Verification items for the finished model (mm, model axes). A direction names the side the tool comes from. Round coordinates to 2 decimals unless told otherwise and drop trailing zeros. Loops run counter-clockwise (first coordinate to the right, second up) from the corner with the lowest first, then second, coordinate; pieces in that order, holes last. Notation, with made-up numbers: (-12, 44) -> (3, 44) arc R17 ccw to (3, 62) -> close; hole circle Ø9 at (-4.5, -38). An arc over 180 degrees is marked (long way). Write item = value, one per line. Start each with the question number.
```python
from build123d import *

# Parameters (mm, degrees)
F0_W     = 11
F0_H     = 22
F0_R     = 0.5
F1_DEPTH = 15
F0_H_2   = 5
F0_R_2   = 1
F2_DEPTH = 1.5
F3_DEPTH = 7


with BuildPart() as f1:
    # F0 (on Top) → F1 (new body)
    with BuildSketch(Plane.XY):
        Rectangle(F0_W, F0_H)
        with Locations((0, -5)):
            Circle(F0_R, mode=Mode.SUBTRACT)
        with Locations((0, -5)):
            Circle(F0_R)
    extrude(amount=F1_DEPTH)

    # F0 (on Top) → F2 (join)
    with BuildSketch(Plane.XY):
        with Locations((0, -13.5)):
            Rectangle(F0_W, F0_H_2)
        with Locations((0, -14.5)):
            Circle(F0_R_2, mode=Mode.SUBTRACT)
        with Locations((0, 13.5)):
            Rectangle(F0_W, F0_H_2)
        with Locations((0, 14.5)):
            Circle(F0_R_2, mode=Mode.SUBTRACT)
    extrude(amount=-F2_DEPTH)

    # F0 (on Top) → F3 (join)
    with BuildSketch(Plane.XY):
        Rectangle(F0_W, F0_H)
        with Locations((0, -5)):
            Circle(F0_R, mode=Mode.SUBTRACT)
    extrude(amount=-F3_DEPTH)


solid = f1.part
```
(1) Section check C-C on y = -5. Enter the section's corners in (x, z), then the cut area to 3 significant figures.
(2) Depth check by flat-ended pin: pin 1 Ø3.5 at (x, z) = (-2, 8.5) entering from +Y; pin 2 Ø0.8 at (x, y) = (0, -5) entering from -Z; pin 3 Ø1.5 at (x, y) = (0.5, -13.5) entering from -Z; pin 4 Ø1.2 at (x, y) = (0, -14.5) entering from -Z. Enter the tip coordinate at first touch or a pass-through.
(3) Section check D-D on x = 1.5. Enter the section's corners in (y, z).
(4) Draft check along X on faces 1 (the cylindrical face through (-0.065, -4.504, -3.451)), 2 (the flat face through (0, -13, -1.5)), 3 (the flat face through (5.5, 0, 4)), 4 (the flat face through (-5.5, 0, 4)). Enter one of: +X half, -X half, draft (parallel to the pull), parting line (faces both ways), or undercut.
(5) Section check A-A on x = 0. Enter the section's corners in (y, z), then the cut area to 3 significant figures.
(6) Access from +Z, -Z, +X, -X, +Y, -Y to the whole of each face (thin tool, end or side, straight path). Record for faces 5 (the flat face through (0, 11, -4)), 6 (the flat face through (0, -11, -4)), 7 (the flat face through (0, -5, 0)), 8 (the flat face through (0, 11, 7)), 9 (the flat face through (0, -11, 7)).
(7) Section check B-B on y = 14.5. Enter the section's corners in (x, z).
(8) Scan lines: line 1 (Y direction, x = 0, z = -0.8); line 2 (Y direction, x = 0, z = -4.25); line 3 (Y direction, x = -3.5, z = -5). Record each from-to range of solid material in increasing order. Write a range as [from, to].
Computed values:
q1.outline = (-5.5, -7) -> (-0.5, -7) -> (-0.5, 0) -> (0.5, 0) -> (0.5, -7) -> (5.5, -7) -> (5.5, 15) -> (-5.5, 15) -> close
q1.area = 235 mm²
q2.pin_1 = 11
q2.pin_2 = 0
q2.pin_3 = -1.5
q2.pin_4 = through
q3.outline = (-16, -1.5) -> (-11, -1.5) -> (-11, -7) -> (11, -7) -> (11, -1.5) -> (16, -1.5) -> (16, 0) -> (11, 0) -> (11, 15) -> (-11, 15) -> (-11, 0) -> (-16, 0) -> close
q4.face_1 = undercut
q4.face_2 = draft
q4.face_3 = +X half
q4.face_4 = -X half
q5.outline = (-16, -1.5) -> (-15.5, -1.5) -> (-15.5, 0) -> (-16, 0) -> close; (-13.5, -1.5) -> (-11, -1.5) -> (-11, -7) -> (-5.5, -7) -> (-5.5, 0) -> (-4.5, 0) -> (-4.5, -7) -> (11, -7) -> (11, -1.5) -> (13.5, -1.5) -> (13.5, 0) -> (11, 0) -> (11, 15) -> (-11, 15) -> (-11, 0) -> (-13.5, 0) -> close; (15.5, -1.5) -> (16, -1.5) -> (16, 0) -> (15.5, 0) -> close
q5.area = 486 mm²
q6.face_5 = -Z, +X, -X, +Y
q6.face_6 = -Z, +X, -X, -Y
q6.face_7 = -Z
q6.face_8 = +Z, +X, -X, +Y
q6.face_9 = +Z, +X, -X, -Y
q7.outline = (-5.5, -1.5) -> (-1, -1.5) -> (-1, 0) -> (-5.5, 0) -> close; (1, -1.5) -> (5.5, -1.5) -> (5.5, 0) -> (1, 0) -> close
q8.line_1 = [-16, -15.5], [-13.5, -5.5], [-4.5, 13.5], [15.5, 16]
q8.line_2 = [-11, -5.5], [-4.5, 11]
q8.line_3 = [-11, 11]
